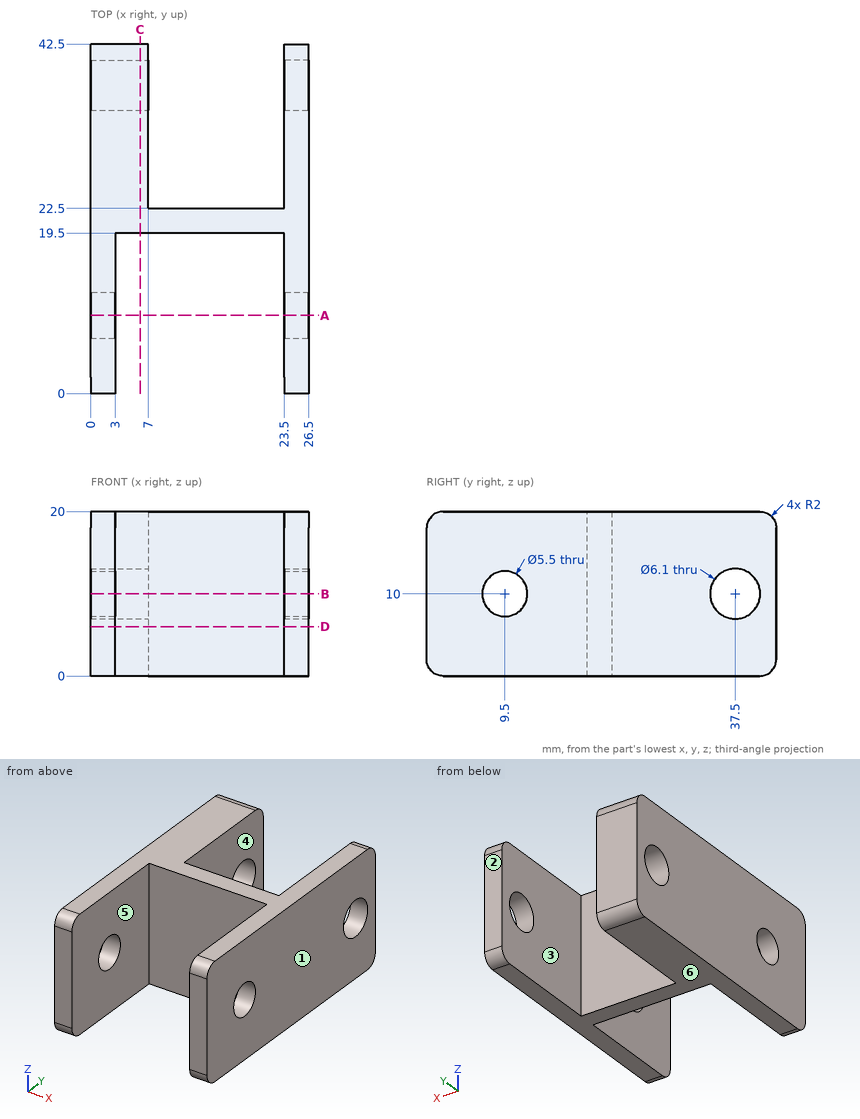
Could you check a few things on this drawing? It's one solid part, dimensions in mm from its lowest x, y, z. A direction names the side the tool comes from. Give positions to 0.01 mm unless a question says otherwise; leave off trailing zeros. Write each loop counter-clockwise with the first axis right and the second up, starting at its lowest first coordinate (ties: lowest second). Pieces come first, ordered by that corner, then holes. Notation, with made-up numbers: (-24.5, -3.5) -> (-8.5, -3.5) arc R32 ccw to (-8.5, 28.5) -> close; hole circle Ø5 at (38, -28). An arc over 180 degrees is marked (long way). Answer as a JSON object with one key per item and string values.
Q1. Will these pins go through, and if not, where does the flat tip stop? pin 1 Ø5 at (x, z) = (8, 7) entering from -Y; pin 2 Ø12 at (y, z) = (18, 10.5) entering from -X; pin 3 Ø8 at (x, z) = (16.5, 10) entering from +Y.
Taken from the geometry:
{"pin 1": "stops at y = 19.5", "pin 2": "stops at x = 0", "pin 3": "stops at y = 22.5"}
Q2. Suppose I cut it at C-C on x = 6. Write out the boundary of the cut face in (y, z), then the cut area to 3 significant figures.
Taken from the geometry:
{"outline": "(19.5, 0) -> (40.5, 0) arc R2 ccw to (42.5, 2) -> (42.5, 18) arc R2 ccw to (40.5, 20) -> (19.5, 20) -> close; hole circle Ø6.1 at (37.5, 10)", "area": "429 mm²"}
Q3. Which directions (+Z, -Z, +X, -X, +Y, -Y) give clear straight access to the entire face, cutting with the end or side of a thin tool? Please do the marked faces 4, 5 and 6.
Taken from the geometry:
{"face 4": "+Z, -Z, +Y", "face 5": "+Z, -Z, -Y", "face 6": "-Z, +X, -X, +Y, -Y"}
Q4. Suppose I cut it at D-D on z = 6. Write out the boundary of the cut face in (x, y).
Taken from the geometry:
{"outline": "(0, 0) -> (3, 0) -> (3, 19.5) -> (23.5, 19.5) -> (23.5, 0) -> (26.5, 0) -> (26.5, 42.5) -> (23.5, 42.5) -> (23.5, 22.5) -> (7, 22.5) -> (7, 42.5) -> (0, 42.5) -> close"}
Q5. Suppose I cut it at A-A on y = 9.5. Write out the boundary of the cut face in (x, z).
Taken from the geometry:
{"outline": "(0, 0) -> (3, 0) -> (3, 7.25) -> (0, 7.25) -> close; (0, 12.75) -> (3, 12.75) -> (3, 20) -> (0, 20) -> close; (23.5, 0) -> (26.5, 0) -> (26.5, 7.25) -> (23.5, 7.25) -> close; (23.5, 12.75) -> (26.5, 12.75) -> (26.5, 20) -> (23.5, 20) -> close"}
Q6. Please list where these lines run through material, in increasing order: L1, parallel to X at y = 6.5, z = 17.75; L2, parallel to Z at x = 24.4, y = 9.5; L3, parallel to X at y = 35, z = 7.5.
Taken from the geometry:
{"L1": "x = 0 to 3, 23.5 to 26.5", "L2": "z = 0 to 7.25, 12.75 to 20", "L3": "x = 0 to 7, 23.5 to 26.5"}
Q7. Suppose I cut it at B-B on z = 10. Write out the boundary of the cut face in (x, y).
Taken from the geometry:
{"outline": "(0, 0) -> (3, 0) -> (3, 6.75) -> (0, 6.75) -> close; (0, 12.25) -> (3, 12.25) -> (3, 19.5) -> (23.5, 19.5) -> (23.5, 12.25) -> (26.5, 12.25) -> (26.5, 34.45) -> (23.5, 34.45) -> (23.5, 22.5) -> (7, 22.5) -> (7, 34.45) -> (0, 34.45) -> close; (0, 40.55) -> (7, 40.55) -> (7, 42.5) -> (0, 42.5) -> close; (23.5, 0) -> (26.5, 0) -> (26.5, 6.75) -> (23.5, 6.75) -> close; (23.5, 40.55) -> (26.5, 40.55) -> (26.5, 42.5) -> (23.5, 42.5) -> close"}
Q8. We'd pull the mould along X, two halves only. Please class the marked faces 1, 2 and 3: released by +X, released by -X, zero draft, split by the parting line, or undercut.
Taken from the geometry:
{"face 1": "released by +X", "face 2": "zero draft", "face 3": "undercut"}
